```python
from build123d import *

# Parameters (mm, degrees)
F0_W         = 277
F0_H         = 197
F1_DEPTH     = 22
F2_W         = 268
F2_H         = 188
F3_DEPTH     = 3.5
F4_T4_DEPTH  = 188
F4_T9_DEPTH  = 268
F4_T14_DEPTH = 188
F4_T19_DEPTH = 268


# Not quite as in the source:
# - a fillet or chamfer that OpenCascade refuses, or shapes differently, is made with other operations: its cross-section is extruded or revolved along the edge and cut away or added


with BuildPart() as f1:
    # F0 (on Top) → F1 (new body)
    with BuildSketch(Plane.XY):
        Rectangle(F0_W, F0_H)
    extrude(amount=F1_DEPTH)

    # F2 (on face) → F3 (cut)
    with BuildSketch(Plane.XY.offset(22)):
        Rectangle(F2_W, F2_H)
    extrude(amount=-F3_DEPTH, mode=Mode.SUBTRACT)

    # F4: chamfer of 4.5 x 3.5157853193 on 4 edges, made by hand


with BuildPart() as f4_tool2:
    # F4_s3 → F4_t4 (new body)
    with BuildSketch(Plane.XZ.offset(94)):
        Polygon((134, 22.0157853193), (129.5, 18.5), (134, 18.5), align=None)
    extrude(amount=-F4_T4_DEPTH)

    split(bisect_by=Plane.XY.offset(22), keep=Keep.BOTTOM)


with BuildPart() as f1_1:
    add(f1.part)

    # F4_t1: union F4_tool2
    add(f4_tool2.part)


with BuildPart() as f4_tool7:
    # F4_s8 → F4_t9 (new body)
    with BuildSketch(Plane.YZ.offset(134)):
        Polygon((94, 22.0157853193), (89.5, 18.5), (94, 18.5), align=None)
    extrude(amount=-F4_T9_DEPTH)

    split(bisect_by=Plane.XY.offset(22), keep=Keep.BOTTOM)


with BuildPart() as f1_2:
    add(f1_1.part)

    # F4_t6: union F4_tool7
    add(f4_tool7.part)


with BuildPart() as f4_tool12:
    # F4_s13 → F4_t14 (new body)
    with BuildSketch(Plane.XZ.offset(-94)):
        Polygon((-134, 22.0157853193), (-129.5, 18.5), (-134, 18.5), align=None)
    extrude(amount=F4_T14_DEPTH)

    split(bisect_by=Plane.XY.offset(22), keep=Keep.BOTTOM)


with BuildPart() as f1_3:
    add(f1_2.part)

    # F4_t11: union F4_tool12
    add(f4_tool12.part)


with BuildPart() as f4_tool17:
    # F4_s18 → F4_t19 (new body)
    with BuildSketch(Plane.YZ.offset(-134)):
        Polygon((-94, 22.0157853193), (-89.5, 18.5), (-94, 18.5), align=None)
    extrude(amount=F4_T19_DEPTH)

    split(bisect_by=Plane.XY.offset(22), keep=Keep.BOTTOM)


with BuildPart() as f1_4:
    add(f1_3.part)

    # F4_t16: union F4_tool17
    add(f4_tool17.part)


solid = f1_4.part
```
Could you check a few things on this model? Use its own coordinates, in mm. Coordinates: 2 decimals unless noted, no trailing zeros. Order: outer loops, then holes, each group sorted by start corner. A loop starts at its lowest first (then second) coordinate and runs counter-clockwise, first axis right, second up. Notation, with made-up numbers: M -21.75,42 L 28.25,42 A24 ccw 28.25,58 Z; hole C -0.5,67.5 d7. An arc over 180 degrees is marked long. Use a Markdown table: item, result. Add a question column.
Q1. I'm going to push flat-ended pins straight in: pin 1 (1.5 mm diameter, centred on x = -59.5, y = -66, fed in from -Z); pin 2 (2 mm diameter, centred on x = 100.5, y = 48.5, fed in from +Z). Where does each tip first touch, or does it pass through?
Q2. I want a section at B-B on x = -118.5. List the corners of the cut face in (y, z) for me.
Q3. If I drill on L1, parallel to Z at x = -121.5, y = -20; L2, parallel to X at y = -85, z = 19; L3, parallel to Z at x = 120, y = 90, over which ranges is the centre line in solid material (lowest first)?
Q4. I want a section at A-A on y = 8.5. List the corners of the cut face in (x, z) for me, then the cut area to 3 significant figures.
Q5. We'd pull the mould along Y, two halves only. Please class faces 1 (the flat face through (138.5, -1, 11)), 2 (the flat face through (-2, 1, 18.5)), 3 (the flat face through (-2, -98.5, 11)): pulls with the +Y half, pulls with the -Y half, needs draft (parallel to the pull), parting line crosses it, or undercut.
Checked values:
| question | item | result |
|---|---|---|
| 1 | pin 1 | z = 0 |
| 1 | pin 2 | z = 18.5 |
| 2 | outline | M -98.5,0 L 98.5,0 L 98.5,22 L 93.98,22 L 89.5,18.5 L -89.5,18.5 L -93.98,22 L -98.5,22 Z |
| 3 | L1 | 0 to 18.5 |
| 3 | L2 | -138.5 to -130.14, 130.14 to 138.5 |
| 3 | L3 | 0 to 18.89 |
| 4 | outline | M -138.5,0 L 138.5,0 L 138.5,22 L 133.98,22 L 129.5,18.5 L -129.5,18.5 L -133.98,22 L -138.5,22 Z |
| 4 | area | 5,170 mm² |
| 5 | face 1 | needs draft |
| 5 | face 2 | undercut |
| 5 | face 3 | pulls with the -Y half |
